Read the model definition and answer for the solid it produces. Units are mm, in the model's axes. Face numbers are marked on the shaded views. A direction names the side the tool comes from. Give positions to 0.01 mm unless a question says otherwise; leave off trailing zeros. Order: outer loops, then holes, each group sorted by start corner. A loop starts at its lowest first (then second) coordinate and runs counter-clockwise, first axis right, second up. Notation, with made-up numbers: (64, 79) - (102, 79) arc R23 cw to (102, 89) - close; hole circle Ø6 at (8.5, 25.25). An arc over 180 degrees is marked (long way). Write each question's results on one line, items separated by ' | '. Start each with the question number.
Q1. For a pull along Z with two mould halves and no side action, classify the marked faces 4, 5 and 6 as +Z half, -Z half, draft (parallel to the pull), parting line (faces both ways), or undercut.
Q2. Find the intervals of material crossed by line 1 along X through (y, z) = (4.25, 0); line 2 along X through (y, z) = (30, 4.75); line 3 along X through (y, z) = (18.6, 2.5), in increasing order. Write a range as from..to.
Q3. Find section D-D on z = 0. Give the vertices of the cut face in (x, y), and give its area (3 significant figures).
Q4. Flat-ended cylindrical pins translate along their axes: P1, Ø2, axis at y = 16.5, z = 5.5, coming from the +X side; P2, Ø5.5, axis at x = -13.5, z = -1.5, coming from the +Y side; P3, Ø10, axis at x = -11.5, y = 33.5, coming from the +Z side; P4, Ø5.5, axis at y = 33, z = 0, coming from the -X side. Find the tip coordinate at first contact, or state that the pin passes through.
Q5. Find section A-A on y = 33. Give the vertices of the cut face in (x, z), and give its area (3 significant figures).
Q6. Find section B-B on x = 16. Give the vertices of the cut face in (y, z).
Q7. Find section C-C on y = 29. Give the vertices of the cut face in (x, z).
Q8. A tool of negligible diameter and unlimited length cuts with its end or side. For the marked faces 1, 2 and 3, from which of +Z, -Z, +X, -X, +Y, -Y can it reach the whole face along a straight path? Write none if from no direction.
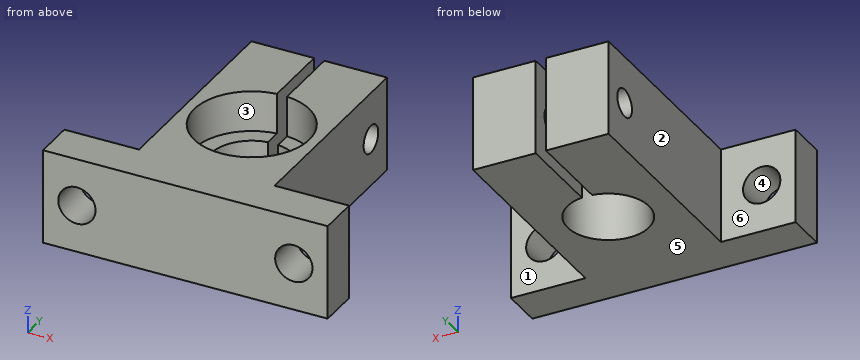
from build123d import *

# Parameters (mm, degrees)
BOSS_EXTRUDE1_DEPTH = 7
SKETCH2_R           = 6
CUT_EXTRUDE1_DEPTH  = 15
SKETCH3_R           = 2.05
CUT_EXTRUDE2_DEPTH  = 32
SKETCH4_R           = 2.75
CUT_EXTRUDE3_DEPTH  = 14
SKETCH5_W           = 1.5
SKETCH5_H           = 29
CUT_EXTRUDE4_DEPTH  = 15
SKETCH6_R           = 8.5
CUT_EXTRUDE5_DEPTH  = 6


with BuildPart() as part:
    # Sketch1 → Boss-Extrude1 (new body, symmetric)
    with BuildSketch(Plane.XY):
        Polygon((0, 0), (21, 0), (21, 6), (10, 6), (10, 37.5), (0, 37.5), align=None)
    boss_extrude1 = extrude(amount=BOSS_EXTRUDE1_DEPTH, both=True)

    # Mirror1: Boss-Extrude1 across plane
    add(boss_extrude1.mirror(Plane(origin=(0, 37.5, 7), x_dir=(0, 0, 1), z_dir=(1, 0, 0))))

    # Sketch2 → Cut-Extrude1 (cut, through all)
    with BuildSketch(Plane.XY.offset(7)):
        with Locations((0, 18.6)):
            Circle(SKETCH2_R)
    extrude(amount=-CUT_EXTRUDE1_DEPTH, mode=Mode.SUBTRACT)

    # Sketch3 → Cut-Extrude2 (cut, through all)
    with BuildSketch(Plane(origin=(10, 0, 0), x_dir=(0, 0, -1), z_dir=(1, 0, 0))):
        with Locations((0, 33)):
            Circle(SKETCH3_R)
    extrude(amount=-CUT_EXTRUDE2_DEPTH, mode=Mode.SUBTRACT)

    # Sketch4 → Cut-Extrude3 (cut)
    with BuildSketch(Plane(origin=(0, 6, 0), x_dir=(1, 0, 0), z_dir=(0, 1, 0))):
        with Locations((-16, 0)):
            Circle(SKETCH4_R)
        with Locations((16, 0)):
            Circle(SKETCH4_R)
    extrude(amount=-CUT_EXTRUDE3_DEPTH, mode=Mode.SUBTRACT)

    # Sketch5 → Cut-Extrude4 (cut, through all)
    with BuildSketch(Plane.XY.offset(7)):
        with Locations((0, 37.5)):
            Rectangle(SKETCH5_W, SKETCH5_H)
    extrude(amount=-CUT_EXTRUDE4_DEPTH, mode=Mode.SUBTRACT)

    # Sketch6 → Cut-Extrude5 (cut)
    with BuildSketch(Plane.XY.offset(7)):
        with Locations((0, 18.6)):
            Circle(SKETCH6_R)
    extrude(amount=-CUT_EXTRUDE5_DEPTH, mode=Mode.SUBTRACT)


solid = part.part
Working result:
1) face 4: undercut | face 5: -Z half | face 6: draft
2) line 1: -21..-18.75, -13.25..13.25, 18.75..21 | line 2: -10..-0.75, 0.75..10 | line 3: -10..-8.5, 8.5..10
3) outline: (-21, 0) - (-18.75, 0) - (-18.75, 6) - (-21, 6) - close; (-13.25, 0) - (13.25, 0) - (13.25, 6) - (10, 6) - (10, 30.95) - (0.75, 30.95) - (0.75, 24.55) arc R6 cw (long way) to (-0.75, 24.55) - (-0.75, 30.95) - (-10, 30.95) - (-10, 6) - (-13.25, 6) - close; (-10, 35.05) - (-0.75, 35.05) - (-0.75, 37.5) - (-10, 37.5) - close; (0.75, 35.05) - (10, 35.05) - (10, 37.5) - (0.75, 37.5) - close; (18.75, 0) - (21, 0) - (21, 6) - (18.75, 6) - close | area: 608 mm²
4) P1: x = 10 | P2: y = 6 | P3: z = 7 | P4: x = -10
5) outline: (-10, -7) - (-0.75, -7) - (-0.75, -2.05) - (-10, -2.05) - close; (-10, 2.05) - (-0.75, 2.05) - (-0.75, 7) - (-10, 7) - close; (0.75, -7) - (10, -7) - (10, -2.05) - (0.75, -2.05) - close; (0.75, 2.05) - (10, 2.05) - (10, 7) - (0.75, 7) - close | area: 183 mm²
6) outline: (0, -7) - (6, -7) - (6, -2.75) - (0, -2.75) - close; (0, 2.75) - (6, 2.75) - (6, 7) - (0, 7) - close
7) outline: (-10, -7) - (-0.75, -7) - (-0.75, 7) - (-10, 7) - close; (0.75, -7) - (10, -7) - (10, 7) - (0.75, 7) - close
8) face 1: +Z, -Z, +X, +Y | face 2: +Z, -Z, -X, +Y | face 3: +Z
